Verification items for this drawing (mm, ordinates from the low corner). Round coordinates to 2 decimals unless told otherwise and drop trailing zeros. Loops run counter-clockwise (first coordinate to the right, second up) from the corner with the lowest first, then second, coordinate; pieces in that order, holes last. Notation, with made-up numbers: M -4,-32 L 31,-32 A25 ccw 31,5 Z; hole C 10,30.5 d5. An arc over 180 degrees is marked long. Answer as CSV lines item,"result".
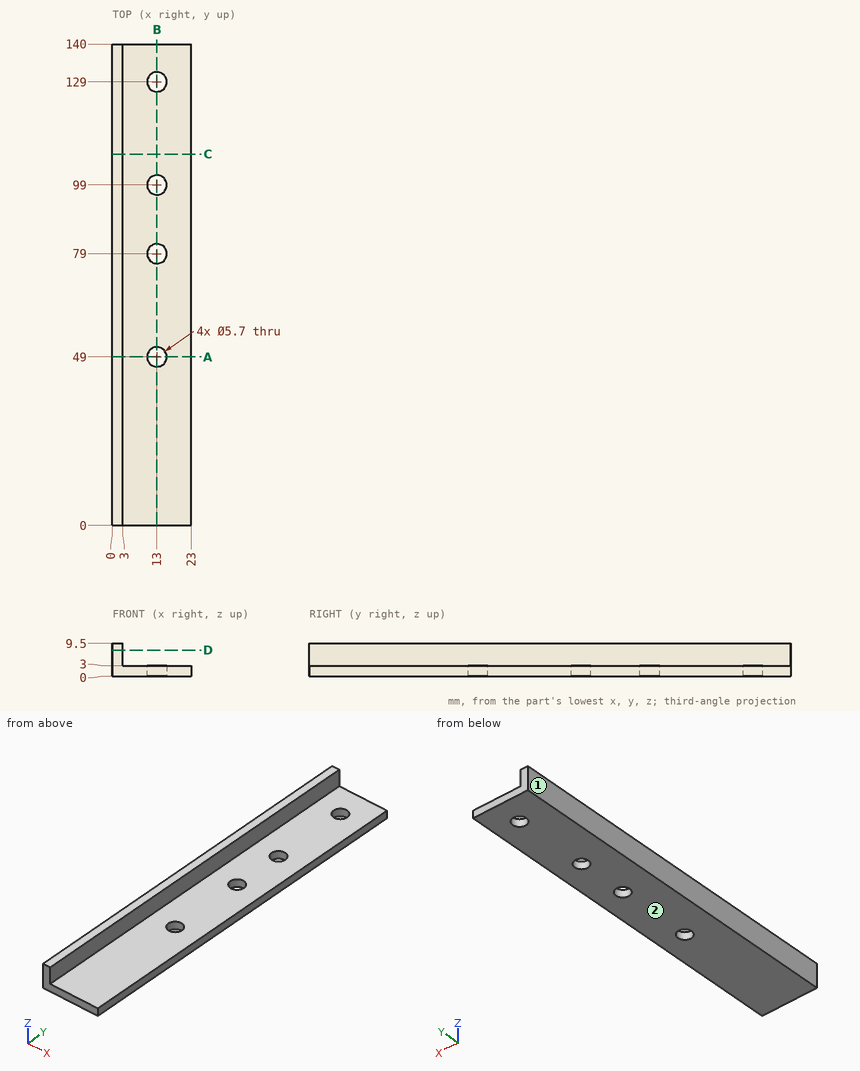
1) Material ranges on probe 1 along Y at (x, z) = (13, 1.05); probe 2 along Z at (x, y) = (21.5, 26.5), recorded low to high.
Here are the results:
probe 1,"y = 0 to 46.15, 51.85 to 76.15, 81.85 to 96.15, 101.85 to 126.15, 131.85 to 140"
probe 2,"z = 0 to 3"
2) Section check D-D (z = 7.5). Record the cut outline in (x, y).
Here are the results:
outline,"M 0,0 L 3,0 L 3,140 L 0,140 Z"
3) Draft check along X on the marked faces 1 and 2. Enter one of: +X half, -X half, draft (parallel to the pull), parting line (faces both ways), or undercut.
Here are the results:
face 1,"-X half"
face 2,"draft"
4) Section check B-B (x = 13). Record the cut outline in (y, z).
Here are the results:
outline,"M 0,0 L 46.15,0 L 46.15,3 L 0,3 Z; M 51.85,0 L 76.15,0 L 76.15,3 L 51.85,3 Z; M 81.85,0 L 96.15,0 L 96.15,3 L 81.85,3 Z; M 101.85,0 L 126.15,0 L 126.15,3 L 101.85,3 Z; M 131.85,0 L 140,0 L 140,3 L 131.85,3 Z"
5) Section check C-C (y = 108). Record the cut outline in (x, z).
Here are the results:
outline,"M 0,0 L 23,0 L 23,3 L 3,3 L 3,9.5 L 0,9.5 Z"
6) Go/stop test with flat-tipped pins: pin 1 (3 mm diameter, centred on x = 19, y = 116.5, fed in from -Z); pin 2 (6 mm diameter, centred on x = 9, y = 21.5, fed in from +Z); pin 3 (3 mm diameter, centred on y = 66, z = 6.5, fed in from +X). Record where each tip stops, or that it passes through.
Here are the results:
pin 1,"stops at z = 0"
pin 2,"stops at z = 3"
pin 3,"stops at x = 3"
7) Section check A-A (y = 49). Record the cut outline in (x, z).
Here are the results:
outline,"M 0,0 L 10.15,0 L 10.15,3 L 3,3 L 3,9.5 L 0,9.5 Z; M 15.85,0 L 23,0 L 23,3 L 15.85,3 Z"
